Source: three-view drawing plus pictorial views. Frame: mm from the lowest corner of the part. Round coordinates to 2 decimals unless told otherwise and drop trailing zeros. Write each loop counter-clockwise with the first axis right and the second up, starting at its lowest first coordinate (ties: lowest second). Pieces come first, ordered by that corner, then holes.
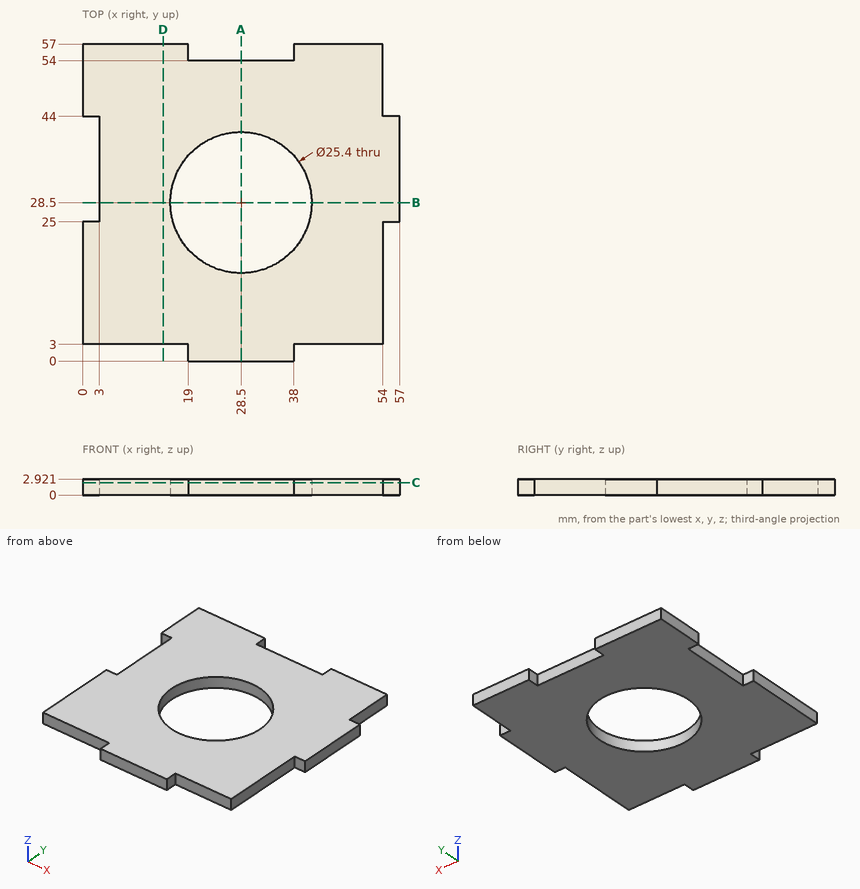
1) Section C-C on z = 2.25. Output: boundary loops of the cut face in (x, y).
2) Section A-A on x = 28.5. Output: boundary loops of the cut face in (y, z).
3) Section B-B on y = 28.5. Output: boundary loops of the cut face in (x, z), plus the area to 3 significant figures.
4) Section D-D on x = 14.5. Output: boundary loops of the cut face in (y, z), plus the area to 3 significant figures.
5) First-contact query: P1, Ø1.5, axis at x = 55, z = 1.5, coming from the +Y side; P2, Ø1.5, axis at y = 1, z = 1.5, coming from the -X side; P3, Ø1.5, axis at x = 2, z = 1.5, coming from the -Y side; P4, Ø1.5, axis at x = 31, y = 18, coming from the -Z side. Flat tips, straight axial feed; report the tip coordinate or a pass-through.
6) Line query: probe 1 along Y at (x, z) = (28.5, 1.65); probe 2 along X at (y, z) = (28.5, 1.1); probe 3 along X at (y, z) = (10, 2.45). Output: solid intervals per line, ascending.
Filled in:
1. outline: (0, 3) - (19, 3) - (19, 0) - (38, 0) - (38, 3) - (54, 3) - (54, 25) - (57, 25) - (57, 44) - (54, 44) - (54, 57) - (38, 57) - (38, 54) - (19, 54) - (19, 57) - (0, 57) - (0, 44) - (3, 44) - (3, 25) - (0, 25) - close; hole circle Ø25.4 at (28.5, 28.5)
2. outline: (0, 0) - (15.8, 0) - (15.8, 2.92) - (0, 2.92) - close; (41.2, 0) - (54, 0) - (54, 2.92) - (41.2, 2.92) - close
3. outline: (3, 0) - (15.8, 0) - (15.8, 2.92) - (3, 2.92) - close; (41.2, 0) - (57, 0) - (57, 2.92) - (41.2, 2.92) - close
3. area: 83.5 mm2
4. outline: (3, 0) - (57, 0) - (57, 2.92) - (3, 2.92) - close
4. area: 158 mm2
5. P1: stops at y = 44
5. P2: stops at x = 19
5. P3: stops at y = 3
5. P4: passes through
6. probe 1: y = 0 to 15.8, 41.2 to 54
6. probe 2: x = 3 to 15.8, 41.2 to 57
6. probe 3: x = 0 to 54
